from build123d import *

# Parameters (mm, degrees)
SKETCH_1_W             = 250
SKETCH_1_H             = 250
EXTRUDE_1_DEPTH        = 10
SKETCH_4_R             = 8
EXTRUDE_2_DEPTH        = 4
SKETCH_6_R             = 1.5
EXTRUDE_3_DEPTH        = 3
PATTERN_LINEAR_1_COUNT = 6
PATTERN_LINEAR_1_PITCH = 30
DRAFT_1_ANGLE          = 30
PATTERN_LINEAR_2_COUNT = 6
PATTERN_LINEAR_2_PITCH = 30
DRAFT_2_ANGLE          = 30
DRAFT_3_ANGLE          = 30
DRAFT_4_ANGLE          = 30
DRAFT_5_ANGLE          = 30
DRAFT_6_ANGLE          = 30


with BuildPart() as part:
    # 草图1 → 凸台-拉伸1 (new body)
    with BuildSketch(Plane.XY):
        with Locations((16.726943942, -49.050632911)):
            Rectangle(SKETCH_1_W, SKETCH_1_H)
    extrude(amount=EXTRUDE_1_DEPTH)

    # 草图4 → 凸台-拉伸2 (add)
    with BuildSketch(Plane(origin=(0, 0, 0), x_dir=(-1, 0, 0), z_dir=(0, 0, -1))):
        with Locations((-24.479358253, -68.79415652)):
            Circle(SKETCH_4_R)
    extrude(amount=EXTRUDE_2_DEPTH)

    # 草图6 → 凸台-拉伸3 (add)
    with BuildSketch(Plane(origin=(0, 0, 0), x_dir=(-1, 0, 0), z_dir=(0, 0, -1))):
        with Locations((-128.994191702, 14.387355328)):
            Circle(SKETCH_6_R)
    extrude_3 = extrude(amount=EXTRUDE_3_DEPTH)

    # 阵列(线性)1: 凸台-拉伸3 ×6
    with Locations(*[(0, -i * PATTERN_LINEAR_1_PITCH, 0) for i in range(1, PATTERN_LINEAR_1_COUNT)]):
        add(extrude_3)

    # 拔模1
    draft_1_faces = [part.faces().sort_by_distance(p)[0] for p in [
        (130.494191702, 14.387355328, -1.5),
    ]]
    draft(draft_1_faces, Plane(origin=(128.994191702, 14.387355328, -3), x_dir=(-1, 0, 0), z_dir=(0, 0, -1)), DRAFT_1_ANGLE)

    # 阵列(线性)2: 凸台-拉伸3 ×6
    with Locations(*[(0, -i * PATTERN_LINEAR_2_PITCH, 0) for i in range(1, PATTERN_LINEAR_2_COUNT)]):
        add(extrude_3)

    # 拔模2
    draft_2_faces = [part.faces().sort_by_distance(p)[0] for p in [
        (130.494191702, -15.612644672, -1.5),
    ]]
    draft(draft_2_faces, Plane(origin=(128.994191702, -15.612644672, -3), x_dir=(-1, 0, 0), z_dir=(0, 0, -1)), DRAFT_2_ANGLE)

    # 拔模3
    draft_3_faces = [part.faces().sort_by_distance(p)[0] for p in [
        (130.494191702, -45.612644672, -1.5),
    ]]
    draft(draft_3_faces, Plane(origin=(128.994191702, -45.612644672, -3), x_dir=(-1, 0, 0), z_dir=(0, 0, -1)), DRAFT_3_ANGLE)

    # 拔模4
    draft_4_faces = [part.faces().sort_by_distance(p)[0] for p in [
        (130.494191702, -75.612644672, -1.5),
    ]]
    draft(draft_4_faces, Plane(origin=(128.994191702, -75.612644672, -3), x_dir=(-1, 0, 0), z_dir=(0, 0, -1)), DRAFT_4_ANGLE)

    # 拔模5
    draft_5_faces = [part.faces().sort_by_distance(p)[0] for p in [
        (130.494191702, -105.612644672, -1.5),
    ]]
    draft(draft_5_faces, Plane(origin=(128.994191702, -105.612644672, -3), x_dir=(-1, 0, 0), z_dir=(0, 0, -1)), DRAFT_5_ANGLE)

    # 拔模6
    draft_6_faces = [part.faces().sort_by_distance(p)[0] for p in [
        (130.494191702, -135.612644672, -1.5),
    ]]
    draft(draft_6_faces, Plane(origin=(128.994191702, -135.612644672, -3), x_dir=(-1, 0, 0), z_dir=(0, 0, -1)), DRAFT_6_ANGLE)


solid = part.part
Geometry: final body of the model. Coordinates: model frame, mm. A direction names the side the tool comes from. Give positions to 0.01 mm unless a question says otherwise; leave off trailing zeros. Write each loop counter-clockwise with the first axis right and the second up, starting at its lowest first coordinate (ties: lowest second). Pieces come first, ordered by that corner, then holes. Notation, with made-up numbers: (71, -38.75) - (116, -38.75) arc R14 ccw to (116, -23.75) - close; hole circle Ø6 at (-30, 22.5). An arc over 180 degrees is marked (long way). Return JSON: item names as keys, results as strings. Group by question number.
1) First-contact query: P1, Ø1.5, axis at x = 128.5, y = -15, coming from the -Z side; P2, Ø4, axis at y = -144, z = -1, coming from the +X side; P3, Ø3, axis at x = -43, y = -98, coming from the -Z side. Flat tips, straight axial feed; report the tip coordinate or a pass-through.
2) Section A-A on y = -9.5. Return the cut outline in (x, z), plus the area to 3 significant figures.
3) Line query: line 1 (Z direction, x = -68, y = -85.5). Output: solid intervals per line, ascending.
4) Set-up query: faces 5 (the flat face through (-108.273, -51, 5)), 6 (the cylindrical face through (25.521, -60.862, -1.972)). Return all of +Z, -Z, +X, -X, +Y, -Y with unobstructed straight access to the full face (end or side cutting, diameter ignored); none if empty.
5) Section B-B on x = 6. Return the cut outline in (y, z), plus the area to 3 significant figures.
6) Mould query, pull axis Y, two halves, no side actions, for faces 1 (the conical face through (130.793, 14.467, -2.479)), 2 (the flat face through (15, -174.051, 5)), 3 (the flat face through (15, -47, 10)), 4 (the flat face through (15, 75.949, 5)). Classes: released by +Y, released by -Y, zero draft, split by the parting line, or undercut.
Filled in:
{
 "1": {"P1": "stops at z = -3", "P2": "stops at x = 141.73", "P3": "stops at z = 0"},
 "2": {"outline": "(-108.27, 0) - (141.73, 0) - (141.73, 10) - (-108.27, 10) - close", "area": "2,500 mm^2"},
 "3": {"line 1": "z = 0 to 10"},
 "4": {"face 5": "+Z, -Z, -X, +Y, -Y", "face 6": "-Z"},
 "5": {"outline": "(-174.05, 0) - (75.95, 0) - (75.95, 10) - (-174.05, 10) - close", "area": "2,500 mm^2"},
 "6": {"face 1": "undercut", "face 2": "released by -Y", "face 3": "zero draft", "face 4": "released by +Y"}
}
